Drawing for the job (mm, zero at the part's lowest x, y, z). A direction names the side the tool comes from. Give positions to 0.01 mm unless a question says otherwise; leave off trailing zeros. Order: outer loops, then holes, each group sorted by start corner. A loop starts at its lowest first (then second) coordinate and runs counter-clockwise, first axis right, second up. Notation, with made-up numbers: M 75.25,43.25 L 108.25,43.25 A4 ccw 108.25,48.25 Z; hole C 56.25,-17 d10. An arc over 180 degrees is marked long. Answer as a JSON object with one key per item and string values.
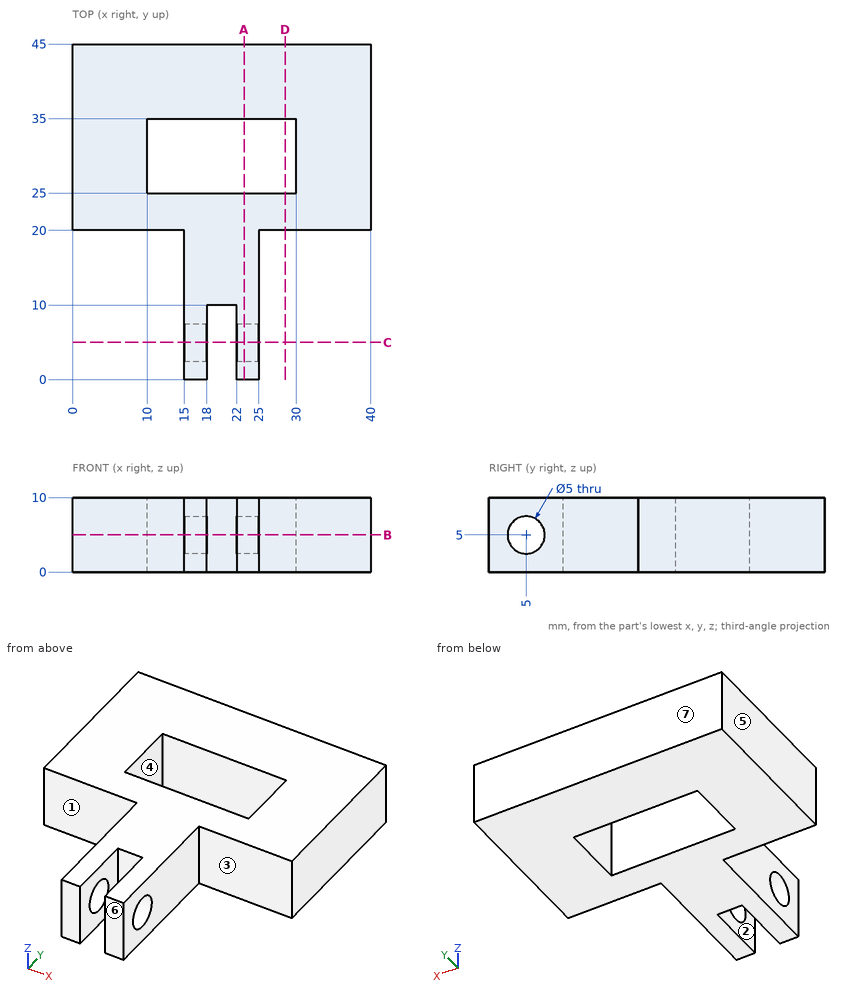
1. Cut at C-C on y = 5. Give the cut face in (x, z).
Worked answers:
{"outline": "M 15,0 L 18,0 L 18,2.5 L 15,2.5 Z; M 15,7.5 L 18,7.5 L 18,10 L 15,10 Z; M 22,0 L 25,0 L 25,2.5 L 22,2.5 Z; M 22,7.5 L 25,7.5 L 25,10 L 22,10 Z"}
2. Two-plate mould, pull along Y, no slides. Class the marked faces 4, 5, 6 and 7: +Y half, -Y half, draft (parallel to the pull), parting line (faces both ways), or undercut.
Worked answers:
{"face 4": "undercut", "face 5": "draft", "face 6": "-Y half", "face 7": "+Y half"}
3. Cut at D-D on x = 28.5. Give the cut face in (y, z), plus the area to 3 significant figures.
Worked answers:
{"outline": "M 20,0 L 25,0 L 25,10 L 20,10 Z; M 35,0 L 45,0 L 45,10 L 35,10 Z", "area": "150 mm^2"}
4. Cut at B-B on z = 5. Give the cut face in (x, y).
Worked answers:
{"outline": "M 0,20 L 15,20 L 15,7.5 L 18,7.5 L 18,10 L 22,10 L 22,7.5 L 25,7.5 L 25,20 L 40,20 L 40,45 L 0,45 Z; M 15,0 L 18,0 L 18,2.5 L 15,2.5 Z; M 22,0 L 25,0 L 25,2.5 L 22,2.5 Z; hole M 10,25 L 30,25 L 30,35 L 10,35 Z"}
5. Cut at A-A on x = 23. Give the cut face in (y, z).
Worked answers:
{"outline": "M 0,0 L 25,0 L 25,10 L 0,10 Z; M 35,0 L 45,0 L 45,10 L 35,10 Z; hole C 5,5 d5"}
6. Pin check, flat tips, straight feed: P1, Ø1.2, axis at x = 19.5, z = 7.5, coming from the -Y side; P2, Ø3, axis at y = 3, z = 4.5, coming from the +X side; P3, Ø3, axis at x = 32, z = 7, coming from the -Y side. Stop position of each tip, or through.
Worked answers:
{"P1": "stops at y = 10", "P2": "stops at x = 25", "P3": "stops at y = 20"}
7. Probe line 1 along Y through (x, z) = (23.7, 5); line 2 along Y through (x, z) = (20.5, 2.75); line 3 along X through (y, z) = (29, 4). List the from-to ranges inside material, lowest first.
Worked answers:
{"line 1": "y = 0 to 2.5, 7.5 to 25, 35 to 45", "line 2": "y = 10 to 25, 35 to 45", "line 3": "x = 0 to 10, 30 to 40"}
8. Which spindle directions (+Z, -Z, +X, -X, +Y, -Y) get a long thin tool onto all of the face, cutting with end or side? Do the marked faces 1, 2 and 3. Say none if no direction does.
Worked answers:
{"face 1": "+Z, -Z, -X, -Y", "face 2": "+Z, -Z, -Y", "face 3": "+Z, -Z, +X, -Y"}
